The drawing under review shows one solid part. Ordinate dimensions are in mm from its lowest x, y, z. Give positions to 0.01 mm unless a question says otherwise; leave off trailing zeros. Order: outer loops, then holes, each group sorted by start corner. A loop starts at its lowest first (then second) coordinate and runs counter-clockwise, first axis right, second up. Notation, with made-up numbers: (52.25, 31) - (107.25, 31) arc R6 ccw to (107.25, 35) - close; hole circle Ø4 at (-19, 55.5). An arc over 180 degrees is marked (long way). Use CSV: the item, a comma, the result in double quotes. Start each with the question number.
1. For pin 1 (3 mm diameter, centred on x = 120, y = 5, fed in from +Z), flat-tipped, find the tip position at first contact; note if it passes through.
2. To check wall thickness, follow line 1 (X direction, y = 5, z = 1.45); line 2 (Y direction, x = 160, z = 3.55); line 3 (Z direction, x = 90, y = 8.75). State the ranges of each line that lie inside material, in increasing order. Write a range as [from, to].
3. Take a section at A-A, the plane z = 3. State the section outline as (x, y) points.
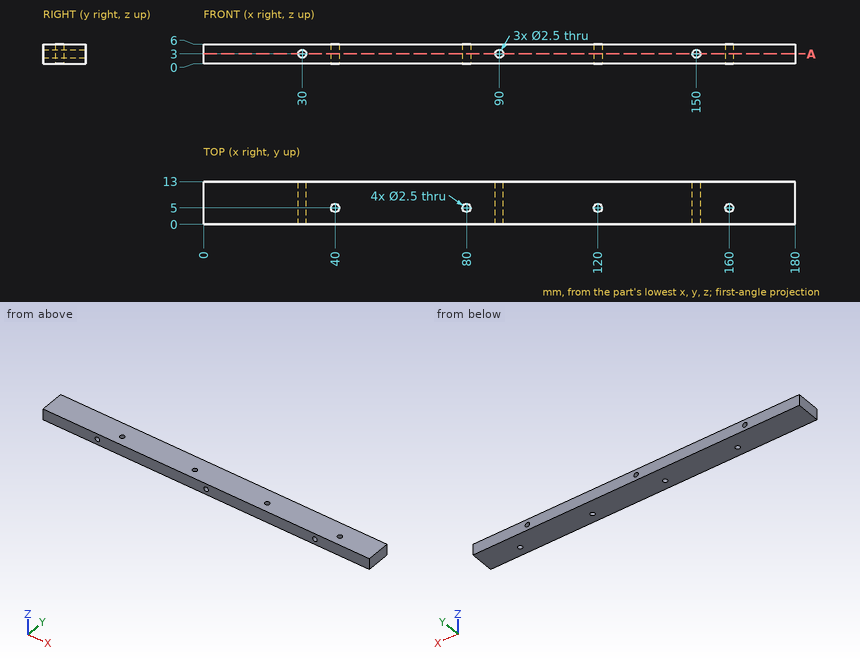
Determined:
1,pin 1,"stops at z = 6"
2,line 1,"x = [0, 38.75], [41.25, 78.75], [81.25, 118.75], [121.25, 158.75], [161.25, 180]"
2,line 2,"y = [0, 3.75], [6.25, 13]"
2,line 3,"z = [0, 1.75], [4.25, 6]"
3,outline,"(0, 0) - (28.75, 0) - (28.75, 13) - (0, 13) - close; (31.25, 0) - (88.75, 0) - (88.75, 13) - (31.25, 13) - close; (91.25, 0) - (148.75, 0) - (148.75, 13) - (91.25, 13) - close; (151.25, 0) - (180, 0) - (180, 13) - (151.25, 13) - close; hole circle Ø2.5 at (40, 5); hole circle Ø2.5 at (80, 5); hole circle Ø2.5 at (120, 5); hole circle Ø2.5 at (160, 5)"
